Source: CAD feature listing. Evaluate the final solid. Frame: model axes, mm. Coordinates: 2 decimals unless noted, no trailing zeros. One line per question, with ' | ' between items. Start each with the question number.
```python
from build123d import *

# Parameters (mm, degrees)
MODEL_R             = 3.175
BOSS_EXTRUDE1_DEPTH = 3.175


with BuildPart() as part:
    # Model → Boss-Extrude1 (new body)
    with BuildSketch(Plane.XY):
        with BuildLine():
            Line((-152.4, -939.8), (-609.6, -939.8))
            ThreePointArc((-609.6, -939.8), (-663.481536726, -962.118463274), (-685.8, -1016))
            Line((-685.8, -1016), (-685.8, -1473.2))
            ThreePointArc((-685.8, -1473.2), (-663.481536726, -1527.081536726), (-609.6, -1549.4))
            Line((-609.6, -1549.4), (-152.4, -1549.4))
            ThreePointArc((-152.4, -1549.4), (-98.518463274, -1527.081536726), (-76.2, -1473.2))
            Line((-76.2, -1473.2), (-76.2, -1016))
            ThreePointArc((-76.2, -1016), (-98.518463274, -962.118463274), (-152.4, -939.8))
        make_face()
        with Locations((-381, -952.5)):
            Circle(MODEL_R, mode=Mode.SUBTRACT)
        with Locations((-88.9, -1473.432930672)):
            Circle(MODEL_R, mode=Mode.SUBTRACT)
        with Locations((-88.9, -1359.132930672)):
            Circle(MODEL_R, mode=Mode.SUBTRACT)
        with Locations((-88.9, -1244.832930672)):
            Circle(MODEL_R, mode=Mode.SUBTRACT)
        with Locations((-88.9, -1130.532930672)):
            Circle(MODEL_R, mode=Mode.SUBTRACT)
        with Locations((-482.6, -1536.7)):
            Circle(MODEL_R, mode=Mode.SUBTRACT)
        with Locations((-584.2, -1536.7)):
            Circle(MODEL_R, mode=Mode.SUBTRACT)
        with Locations((-673.1, -1244.832930672)):
            Circle(MODEL_R, mode=Mode.SUBTRACT)
        with Locations((-279.4, -952.5)):
            Circle(MODEL_R, mode=Mode.SUBTRACT)
        with Locations((-482.6, -952.5)):
            Circle(MODEL_R, mode=Mode.SUBTRACT)
        with Locations((-584.2, -952.5)):
            Circle(MODEL_R, mode=Mode.SUBTRACT)
        with Locations((-177.8, -952.5)):
            Circle(MODEL_R, mode=Mode.SUBTRACT)
        with Locations((-88.9, -1016.232930672)):
            Circle(MODEL_R, mode=Mode.SUBTRACT)
        with Locations((-673.1, -1016.232930672)):
            Circle(MODEL_R, mode=Mode.SUBTRACT)
        with Locations((-673.1, -1130.532930672)):
            Circle(MODEL_R, mode=Mode.SUBTRACT)
        with Locations((-673.1, -1473.432930672)):
            Circle(MODEL_R, mode=Mode.SUBTRACT)
        with Locations((-381, -1536.7)):
            Circle(MODEL_R, mode=Mode.SUBTRACT)
        with Locations((-279.4, -1536.7)):
            Circle(MODEL_R, mode=Mode.SUBTRACT)
        with Locations((-177.8, -1536.7)):
            Circle(MODEL_R, mode=Mode.SUBTRACT)
        with Locations((-673.1, -1359.132930672)):
            Circle(MODEL_R, mode=Mode.SUBTRACT)
    extrude(amount=BOSS_EXTRUDE1_DEPTH)


solid = part.part
```
(1) Cut plane A-A, the plane z = 2.6. State how many separate pieces and enclosed holes the cut face has, and give its area (3 significant figures).
(2) Ray query, L1, parallel to Y at x = -584.2, z = 1.65 (3 decimals); L2, parallel to X at y = -952.5, z = 1.05 (3 decimals); L3, parallel to Y at x = -88.9, z = 0.95. Return the intervals inside material, ascending.
(3) Contact query for a flat-ended pin moving along its axis: pin 1 Ø5.5 at (x, y) = (-381, -1536.7) entering from +Z. Output: stop coordinate, or through.
Here are the results:
1) separate pieces: 1 | enclosed holes: 20 | area: 366,000 mm2
2) L1: y = -1549.4 to -1539.875, -1533.525 to -955.675, -949.325 to -939.8 | L2: x = -651.721 to -587.375, -581.025 to -485.775, -479.425 to -384.175, -377.825 to -282.575, -276.225 to -180.975, -174.625 to -110.279 | L3: y = -1515.32 to -1476.61, -1470.26 to -1362.31, -1355.96 to -1248.01, -1241.66 to -1133.71, -1127.36 to -1019.41, -1013.06 to -973.88
3) pin 1: passes through
